```python
from build123d import *

# Parameters (mm, degrees)
ESQUISSE1_R             = 1.5
BOSS_EXTRU_1_DEPTH      = 7
ESQUISSE2_R             = 5.1
ENL_V_MAT_EXTRU_1_DEPTH = 3.5
ESQUISSE3_R             = 3.25
ENL_V_MAT_EXTRU_2_DEPTH = 4.5


with BuildPart() as part:
    # Esquisse1 → Boss.-Extru.1 (new body)
    with BuildSketch(Plane(origin=(7, 0, 0), x_dir=(0, 0, -1), z_dir=(1, 0, 0))):
        with BuildLine():
            ThreePointArc((-6.728643397, 0.523792937), (-6.749, 0), (-6.728643397, -0.523792937))
            ThreePointArc((-6.728643397, -0.523792937), (-7.89518869, -0.821876255), (-8.869006051, -1.529944991))
            ThreePointArc((-8.869006051, -1.529944991), (-8.827067524, -1.755812898), (-8.779377764, -1.980536814))
            ThreePointArc((-8.779377764, -1.980536814), (-7.608721662, -2.262043257), (-6.416902795, -2.091018776))
            ThreePointArc((-6.416902795, -2.091018776), (-6.235262965, -2.582730485), (-6.016009037, -3.058861924))
            ThreePointArc((-6.016009037, -3.058861924), (-6.97968481, -3.780672557), (-7.608408563, -4.80750654))
            ThreePointArc((-7.608408563, -4.80750654), (-7.483226511, -5.000132097), (-7.353168799, -5.189499843))
            ThreePointArc((-7.353168799, -5.189499843), (-6.163895735, -5.001587189), (-5.128246912, -4.387491836))
            ThreePointArc((-5.128246912, -4.387491836), (-4.772263666, -4.772263666), (-4.387491836, -5.128246912))
            ThreePointArc((-4.387491836, -5.128246912), (-5.001587189, -6.163895735), (-5.189499843, -7.353168799))
            ThreePointArc((-5.189499843, -7.353168799), (-5.000132097, -7.483226511), (-4.80750654, -7.608408563))
            ThreePointArc((-4.80750654, -7.608408563), (-3.780672557, -6.97968481), (-3.058861924, -6.016009037))
            ThreePointArc((-3.058861924, -6.016009037), (-2.582730485, -6.235262965), (-2.091018776, -6.416902795))
            ThreePointArc((-2.091018776, -6.416902795), (-2.262043257, -7.608721662), (-1.980536814, -8.779377764))
            ThreePointArc((-1.980536814, -8.779377764), (-1.755812898, -8.827067524), (-1.529944991, -8.869006051))
            ThreePointArc((-1.529944991, -8.869006051), (-0.821876255, -7.89518869), (-0.523792937, -6.728643397))
            ThreePointArc((-0.523792937, -6.728643397), (0, -6.749), (0.523792937, -6.728643397))
            ThreePointArc((0.523792937, -6.728643397), (0.821876255, -7.89518869), (1.529944991, -8.869006051))
            ThreePointArc((1.529944991, -8.869006051), (1.755812898, -8.827067524), (1.980536814, -8.779377764))
            ThreePointArc((1.980536814, -8.779377764), (2.262043257, -7.608721662), (2.091018776, -6.416902795))
            ThreePointArc((2.091018776, -6.416902795), (2.582730485, -6.235262965), (3.058861924, -6.016009037))
            ThreePointArc((3.058861924, -6.016009037), (3.780672557, -6.97968481), (4.80750654, -7.608408563))
            ThreePointArc((4.80750654, -7.608408563), (5.000132097, -7.483226511), (5.189499843, -7.353168799))
            ThreePointArc((5.189499843, -7.353168799), (5.001587189, -6.163895735), (4.387491836, -5.128246912))
            ThreePointArc((4.387491836, -5.128246912), (4.772263666, -4.772263666), (5.128246912, -4.387491836))
            ThreePointArc((5.128246912, -4.387491836), (6.163895735, -5.001587189), (7.353168799, -5.189499843))
            ThreePointArc((7.353168799, -5.189499843), (7.483226511, -5.000132097), (7.608408563, -4.80750654))
            ThreePointArc((7.608408563, -4.80750654), (6.97968481, -3.780672557), (6.016009037, -3.058861924))
            ThreePointArc((6.016009037, -3.058861924), (6.235262965, -2.582730485), (6.416902795, -2.091018776))
            ThreePointArc((6.416902795, -2.091018776), (7.608721662, -2.262043257), (8.779377764, -1.980536814))
            ThreePointArc((8.779377764, -1.980536814), (8.827067524, -1.755812898), (8.869006051, -1.529944991))
            ThreePointArc((8.869006051, -1.529944991), (7.89518869, -0.821876255), (6.728643397, -0.523792937))
            ThreePointArc((6.728643397, -0.523792937), (6.749, 0), (6.728643397, 0.523792937))
            ThreePointArc((6.728643397, 0.523792937), (7.89518869, 0.821876255), (8.869006051, 1.529944991))
            ThreePointArc((8.869006051, 1.529944991), (8.827067524, 1.755812898), (8.779377764, 1.980536814))
            ThreePointArc((8.779377764, 1.980536814), (7.608721662, 2.262043257), (6.416902795, 2.091018776))
            ThreePointArc((6.416902795, 2.091018776), (6.235262965, 2.582730485), (6.016009037, 3.058861924))
            ThreePointArc((6.016009037, 3.058861924), (6.97968481, 3.780672557), (7.608408563, 4.80750654))
            ThreePointArc((7.608408563, 4.80750654), (7.483226511, 5.000132097), (7.353168799, 5.189499843))
            ThreePointArc((7.353168799, 5.189499843), (6.163895735, 5.001587189), (5.128246912, 4.387491836))
            ThreePointArc((5.128246912, 4.387491836), (4.772263666, 4.772263666), (4.387491836, 5.128246912))
            ThreePointArc((4.387491836, 5.128246912), (5.001587189, 6.163895735), (5.189499843, 7.353168799))
            ThreePointArc((5.189499843, 7.353168799), (5.000132097, 7.483226511), (4.80750654, 7.608408563))
            ThreePointArc((4.80750654, 7.608408563), (3.780672557, 6.97968481), (3.058861924, 6.016009037))
            ThreePointArc((3.058861924, 6.016009037), (2.582730485, 6.235262965), (2.091018776, 6.416902795))
            ThreePointArc((2.091018776, 6.416902795), (2.262043257, 7.608721662), (1.980536814, 8.779377764))
            ThreePointArc((1.980536814, 8.779377764), (1.755812898, 8.827067524), (1.529944991, 8.869006051))
            ThreePointArc((1.529944991, 8.869006051), (0.821876255, 7.89518869), (0.523792937, 6.728643397))
            ThreePointArc((0.523792937, 6.728643397), (0, 6.749), (-0.523792937, 6.728643397))
            ThreePointArc((-0.523792937, 6.728643397), (-0.821876255, 7.89518869), (-1.529944991, 8.869006051))
            ThreePointArc((-1.529944991, 8.869006051), (-1.755812898, 8.827067524), (-1.980536814, 8.779377764))
            ThreePointArc((-1.980536814, 8.779377764), (-2.262043257, 7.608721662), (-2.091018776, 6.416902795))
            ThreePointArc((-2.091018776, 6.416902795), (-2.582730485, 6.235262965), (-3.058861924, 6.016009037))
            ThreePointArc((-3.058861924, 6.016009037), (-3.780672557, 6.97968481), (-4.80750654, 7.608408563))
            ThreePointArc((-4.80750654, 7.608408563), (-5.000132097, 7.483226511), (-5.189499843, 7.353168799))
            ThreePointArc((-5.189499843, 7.353168799), (-5.001587189, 6.163895735), (-4.387491836, 5.128246912))
            ThreePointArc((-4.387491836, 5.128246912), (-4.772263666, 4.772263666), (-5.128246912, 4.387491836))
            ThreePointArc((-5.128246912, 4.387491836), (-6.163895735, 5.001587189), (-7.353168799, 5.189499843))
            ThreePointArc((-7.353168799, 5.189499843), (-7.483226511, 5.000132097), (-7.608408563, 4.80750654))
            ThreePointArc((-7.608408563, 4.80750654), (-6.97968481, 3.780672557), (-6.016009037, 3.058861924))
            ThreePointArc((-6.016009037, 3.058861924), (-6.235262965, 2.582730485), (-6.416902795, 2.091018776))
            ThreePointArc((-6.416902795, 2.091018776), (-7.608721662, 2.262043257), (-8.779377764, 1.980536814))
            ThreePointArc((-8.779377764, 1.980536814), (-8.827067524, 1.755812898), (-8.869006051, 1.529944991))
            ThreePointArc((-8.869006051, 1.529944991), (-7.89518869, 0.821876255), (-6.728643397, 0.523792937))
        make_face()
        Circle(ESQUISSE1_R, mode=Mode.SUBTRACT)
    extrude(amount=-BOSS_EXTRU_1_DEPTH)

    # Esquisse2 → Enlèv. mat.-Extru.1 (cut)
    with BuildSketch(Plane(origin=(7, 0, 0), x_dir=(0, 0, -1), z_dir=(1, 0, 0))):
        Circle(ESQUISSE2_R)
    extrude(amount=-ENL_V_MAT_EXTRU_1_DEPTH, mode=Mode.SUBTRACT)

    # Esquisse3 → Enlèv. mat.-Extru.2 (cut, through all)
    with BuildSketch(Plane(origin=(3.5, 0, 0), x_dir=(0, 0, -1), z_dir=(1, 0, 0))):
        Circle(ESQUISSE3_R)
    extrude(amount=-ENL_V_MAT_EXTRU_2_DEPTH, mode=Mode.SUBTRACT)


solid = part.part
```
Geometry: final body of the model. Coordinates: model frame, mm. A direction names the side the tool comes from. Coordinates: 2 decimals unless noted, no trailing zeros. Loops run counter-clockwise (first coordinate to the right, second up) from the corner with the lowest first, then second, coordinate; pieces in that order, holes last. Notation, with made-up numbers: (61.25, 6) -> (106.25, 6) arc R15 ccw to (106.25, 27) -> close; hole circle Ø5 at (-30.75, 79). An arc over 180 degrees is marked (long way). Use a Markdown table: item, result. Add a question column.
(1) Pin query (flat end, axial travel): pin 1 Ø4 at (x, z) = (5, 6.5) entering from +Y; pin 2 Ø1 at (x, y) = (2.5, -1.5) entering from -Z; pin 3 Ø3 at (y, z) = (-2.5, -2) entering from +X. Return the tip coordinate at first contact, or that it passes through.
(2) Section query C-C, the plane z = -7. Return loops of the section in (x, y).
(3) Access query for faces 3 (the cylindrical face through (3.55, 6.97, 3.77)), 4 (the cylindrical face through (5.3, -4.5, -2.4)), 5 (the cylindrical face through (3.549, -7.88, -0.815)), 6 (the cylindrical face through (3.549, -6.238, -2.576)), 7 (the cylindrical face through (3.55, 3.77, -6.97)). Directions: +Z, -Z, +X, -X, +Y, -Y. A direction counts if a zero-diameter tool reaches every point of the face in a straight line with its end or side. Return the directions, or none.
(4) Line query: line 1 along Y through (x, z) = (2.25, -7); line 2 along Y through (x, z) = (5.5, -6.5); line 3 along X through (y, z) = (0.75, -4.75). Output: solid intervals per line, ascending.
(5) Section query A-A, the plane y = 0. Return loops of the section in (x, z).
(6) Mould query, pull axis Z, two halves, no side actions, for faces 1 (the cylindrical face through (3.549, 7.88, 0.815)), 2 (the cylindrical face through (3.55, -3.79, -6.99)). Classes: pulls with the +Z half, pulls with the -Z half, needs draft (parallel to the pull), parting line crosses it, or undercut.
Answer:
| question | item | result |
|---|---|---|
| 1 | pin 1 | stops at y = 7.61 |
| 1 | pin 2 | stops at z = -8.87 |
| 1 | pin 3 | stops at x = 3.5 |
| 2 | outline | (0, -5.18) -> (7, -5.18) -> (7, -3.8) -> (0, -3.8) -> close; (0, -2.23) -> (7, -2.23) -> (7, -0.55) -> (0, -0.55) -> close; (0, 0.55) -> (7, 0.55) -> (7, 2.23) -> (0, 2.23) -> close; (0, 3.8) -> (7, 3.8) -> (7, 5.18) -> (0, 5.18) -> close |
| 3 | face 3 | +X, -X, +Y |
| 3 | face 4 | +X |
| 3 | face 5 | +X, -X, -Y |
| 3 | face 6 | +X, -X |
| 3 | face 7 | -Z, +X, -X |
| 4 | line 1 | y = -5.18 to -3.8, -2.23 to -0.55, 0.55 to 2.23, 3.8 to 5.18 |
| 4 | line 2 | y = -5.1 to -3.35, -2.12 to 2.12, 3.35 to 5.1 |
| 4 | line 3 | x = 0 to 3.5 |
| 5 | outline | (0, -6.75) -> (7, -6.75) -> (7, -5.1) -> (3.5, -5.1) -> (3.5, -3.25) -> (0, -3.25) -> close; (0, 3.25) -> (3.5, 3.25) -> (3.5, 5.1) -> (7, 5.1) -> (7, 6.75) -> (0, 6.75) -> close |
| 6 | face 1 | undercut |
| 6 | face 2 | pulls with the -Z half |
